Source: three-view drawing plus pictorial views. Frame: mm from the lowest corner of the part. A direction names the side the tool comes from. Give positions to 0.01 mm unless a question says otherwise; leave off trailing zeros. Loops run counter-clockwise (first coordinate to the right, second up) from the corner with the lowest first, then second, coordinate; pieces in that order, holes last. Notation, with made-up numbers: (35, 20) - (56, 20) arc R10 ccw to (56, 38) - close; hole circle Ø9 at (-17, 27). An arc over 180 degrees is marked (long way). Answer in a Markdown table with one row per item.
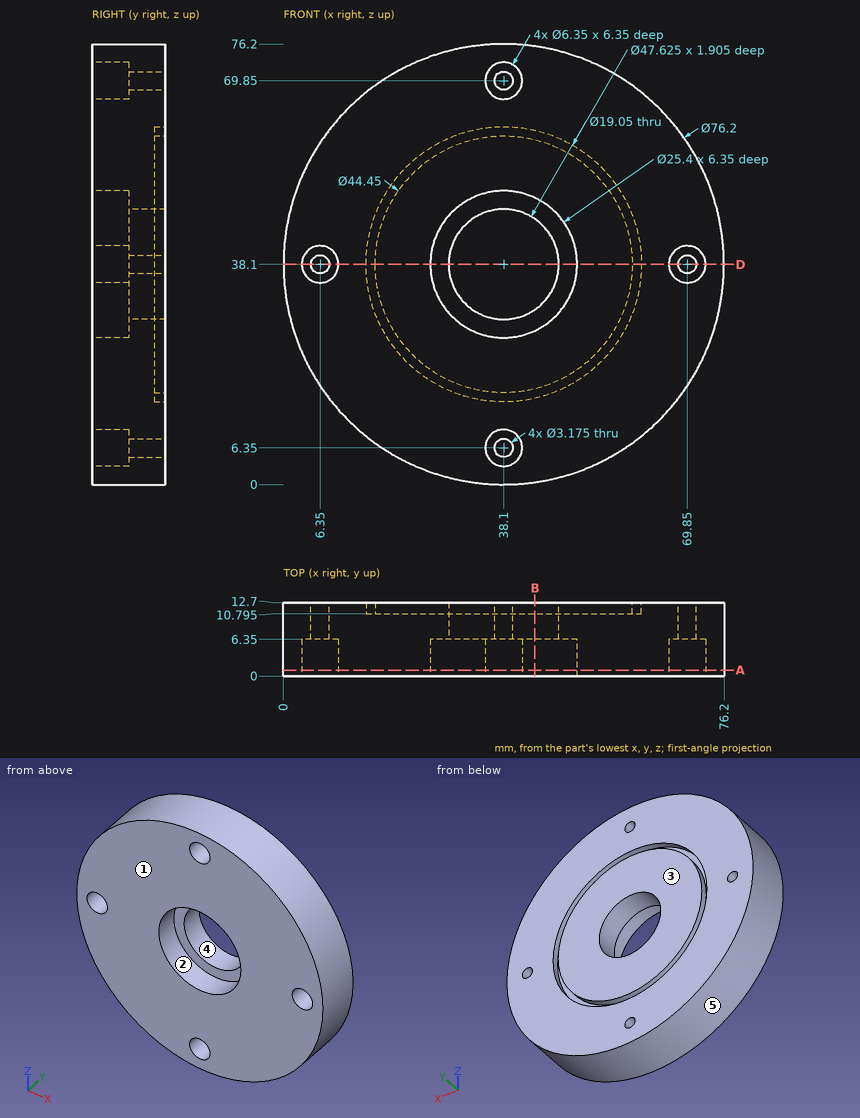
Q1. Cut plane D-D (z = 38.1). Give the number of separate pieces and of enclosed holes in the cut face, and give its area (3 significant figures).
Check values:
| item | result |
|---|---|
| separate pieces | 4 |
| enclosed holes | 0 |
| area | 558 mm² |
Q2. Cut plane B-B (x = 43.5). Output: boundary loops of the cut face in (y, z) (3 decimals).
Check values:
| item | result |
|---|---|
| outline | (0, 0.385) - (12.7, 0.385) - (12.7, 14.908) - (10.795, 14.908) - (10.795, 16.541) - (12.7, 16.541) - (12.7, 30.254) - (6.35, 30.254) - (6.35, 26.605) - (0, 26.605) - close; (0, 49.595) - (6.35, 49.595) - (6.35, 45.946) - (12.7, 45.946) - (12.7, 59.659) - (10.795, 59.659) - (10.795, 61.292) - (12.7, 61.292) - (12.7, 75.815) - (0, 75.815) - close |
Q3. Reachability of the marked faces 1 and 2 from +Z, -Z, +X, -X, +Y, -Y: full face, straight path, thin tool, end or side. Return the list, or none.
Check values:
| item | result |
|---|---|
| face 1 | +Z, -Z, +X, -X, -Y |
| face 2 | -Y |
Q4. Material intervals for line 1 along X through (y, z) = (2.5, 37); line 2 along X through (y, z) = (5.75, 40); line 3 along Z through (x, y) = (5.5, 10.75), sorted ascending.
Check values:
| item | result |
|---|---|
| line 1 | 0.02 to 3.37, 9.33 to 25.45, 50.75 to 66.87, 72.83 to 76.18 |
| line 2 | 0.05 to 3.81, 8.89 to 25.54, 50.66 to 67.31, 72.39 to 76.15 |
| line 3 | 18.38 to 36.76, 39.44 to 57.82 |
Q5. Draft query along Z for the marked faces 3, 4 and 5. Return one class per face: pulls with the +Z half, pulls with the -Z half, needs draft (parallel to the pull), parting line crosses it, or undercut.
Check values:
| item | result |
|---|---|
| face 3 | needs draft |
| face 4 | undercut |
| face 5 | parting line crosses it |
Q6. First-contact query: pin 1 (3 mm diameter, centred on x = 69.85, z = 38.1, fed in from +Y); pin 2 (5 mm diameter, centred on x = 38.1, z = 69.85, fed in from -Y); pin 3 (4 mm diameter, centred on x = 32.5, y = 2.5, fed in from +Z); pin 4 (1 mm diameter, centred on y = 5.5, z = 16, fed in from +X). Flat tips, straight axial feed; report the tip coordinate or a pass-through.
Check values:
| item | result |
|---|---|
| pin 1 | through |
| pin 2 | y = 6.35 |
| pin 3 | z = 76.03 |
| pin 4 | x = 69.49 |
Q7. Cut plane A-A (y = 1). Output: boundary loops of the cut face in (x, z) (3 decimals).
Check values:
| item | result |
|---|---|
| outline | circle Ø76.2 at (38.1, 38.1); hole circle Ø6.35 at (6.35, 38.1); hole circle Ø25.4 at (38.1, 38.1); hole circle Ø6.35 at (38.1, 6.35); hole circle Ø6.35 at (38.1, 69.85); hole circle Ø6.35 at (69.85, 38.1) |
